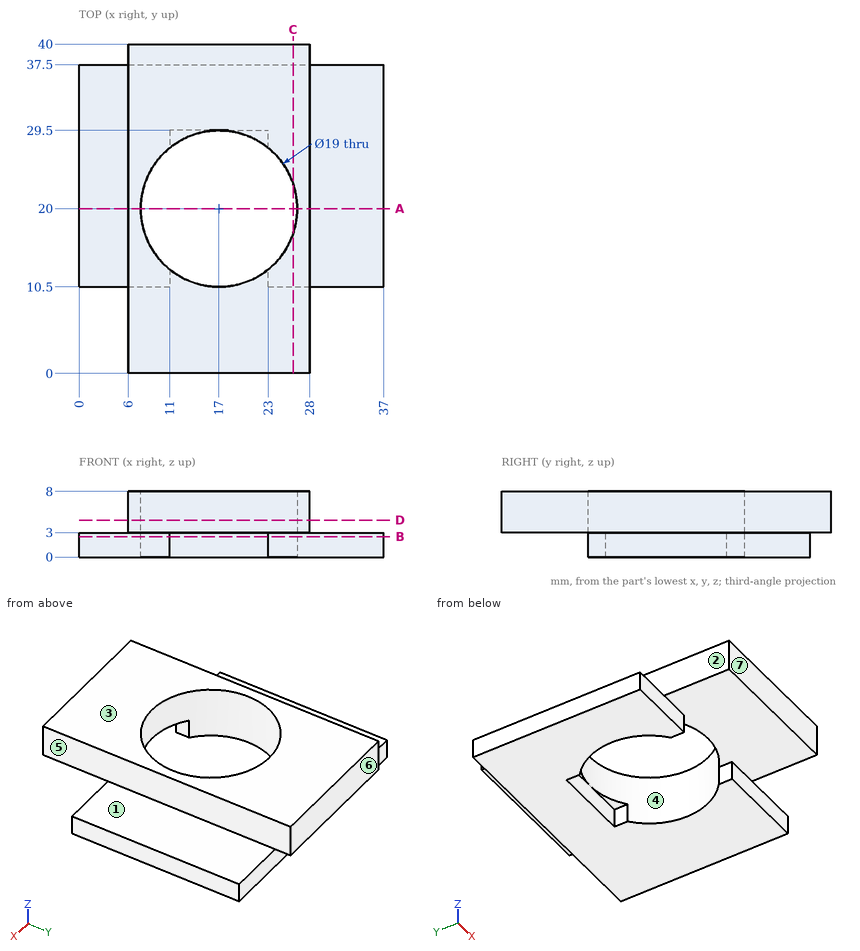
Geometry check sheet. Reference: drawing and pictorial views, mm from the part's lowest x, y, z. A direction names the side the tool comes from. Coordinates: 2 decimals unless noted, no trailing zeros. Order: outer loops, then holes, each group sorted by start corner. A loop starts at its lowest first (then second) coordinate and runs counter-clockwise, first axis right, second up.
Item 1: Depth check by flat-ended pin: pin 1 (2 mm diameter, centred on x = 7.5, z = 2.5, fed in from -Y); pin 2 (0.9 mm diameter, centred on x = 6.5, z = 2, fed in from -Y); pin 3 (4.5 mm diameter, centred on x = 31.5, y = 23.5, fed in from +Z); pin 4 (10 mm diameter, centred on x = 14.5, y = 3.5, fed in from -Z). Enter the tip coordinate at first touch or a pass-through.
Filled in:
pin 1: stops at y = 0
pin 2: stops at y = 10.5
pin 3: stops at z = 3
pin 4: stops at z = 3
Item 2: Section check B-B, the plane z = 2.5. Enter the section's corners in (x, y), then the cut area to 3 significant figures.
Filled in:
outline: (0, 10.5) - (11, 10.5) - (11, 12.63) arc R9.5 cw to (11, 27.37) - (11, 29.5) - (23, 29.5) - (23, 27.37) arc R9.5 cw to (23, 12.63) - (23, 10.5) - (37, 10.5) - (37, 37.5) - (0, 37.5) - close
area: 699 mm2
Item 3: Section check A-A, the plane y = 20. Enter the section's corners in (x, z).
Filled in:
outline: (0, 0) - (7.5, 0) - (7.5, 8) - (6, 8) - (6, 3) - (0, 3) - close; (26.5, 0) - (37, 0) - (37, 3) - (28, 3) - (28, 8) - (26.5, 8) - close
Item 4: Material ranges on L1, parallel to X at y = 20, z = 6.25; L2, parallel to X at y = 20, z = 2.5; L3, parallel to Y at x = 17, z = 5, recorded low to high.
Filled in:
L1: x = 6 to 7.5, 26.5 to 28
L2: x = 0 to 7.5, 26.5 to 37
L3: y = 0 to 10.5, 29.5 to 40
Item 5: Release check for a two-part mould opening along Y. For the marked faces 4, 5, 6 and 7 record: +Y half, -Y half, draft (parallel to the pull), parting line (faces both ways), or undercut.
Filled in:
face 4: undercut
face 5: draft
face 6: +Y half
face 7: -Y half
Item 6: Section check D-D, the plane z = 4.5. Enter the section's corners in (x, y).
Filled in:
outline: (6, 0) - (28, 0) - (28, 40) - (6, 40) - close; hole circle Ø19 at (17, 20)
Item 7: Access from +Z, -Z, +X, -X, +Y, -Y to the whole of each face (thin tool, end or side, straight path). Record for the marked faces 1, 2 and 3.
Filled in:
face 1: +Z, +X, +Y, -Y
face 2: +Z, -X, +Y, -Y
face 3: +Z, +X, -X, +Y, -Y
Item 8: Section check C-C, the plane x = 26. Enter the section's corners in (y, z), then the cut area to 3 significant figures.
Filled in:
outline: (0, 3) - (10.5, 3) - (10.5, 0) - (16.96, 0) - (16.96, 8) - (0, 8) - close; (23.04, 0) - (37.5, 0) - (37.5, 3) - (40, 3) - (40, 8) - (23.04, 8) - close
area: 232 mm2
